from build123d import *

# Parameters (mm, degrees)
F0_W     = 945
F0_H     = 1805
F0_W_2   = 845
F0_H_2   = 1705
F1_DEPTH = 450
F2_W     = 945
F2_H     = 1805
F3_DEPTH = 1
F4_W     = 422.5
F4_H     = 50
F5_DEPTH = 350


with BuildPart() as f1:
    # F0 (on Front) → F1 (new body)
    with BuildSketch(Plane.XZ):
        Rectangle(F0_W, F0_H)
        Rectangle(F0_W_2, F0_H_2, mode=Mode.SUBTRACT)
    extrude(amount=F1_DEPTH)

    # F2 (on face) → F3 (join)
    with BuildSketch(Plane(origin=(0, 0, 0), x_dir=(-1, 0, 0), z_dir=(0, 1, 0))):
        Rectangle(F2_W, F2_H)
    extrude(amount=F3_DEPTH)

    # F4 (on face) → F5 (join)
    with BuildSketch(Plane.XZ):
        Polygon((422.5, 672.5), (-422.5, 672.5), (-422.5, 622.5), (0, 622.5), (50, 622.5), (422.5, 622.5), align=None)
        Polygon((50, 622.5), (0, 622.5), (0, 322.5), (0, 272.5), (0, -27.5), (0, -77.5), (0, -377.5), (0, -427.5), (0, -852.5), (50, -852.5), align=None)
        with Locations((-211.25, 297.5)):
            Rectangle(F4_W, F4_H)
        with Locations((-211.25, -52.5)):
            Rectangle(F4_W, F4_H)
        with Locations((-211.25, -402.5)):
            Rectangle(F4_W, F4_H)
    extrude(amount=F5_DEPTH)


solid = f1.part
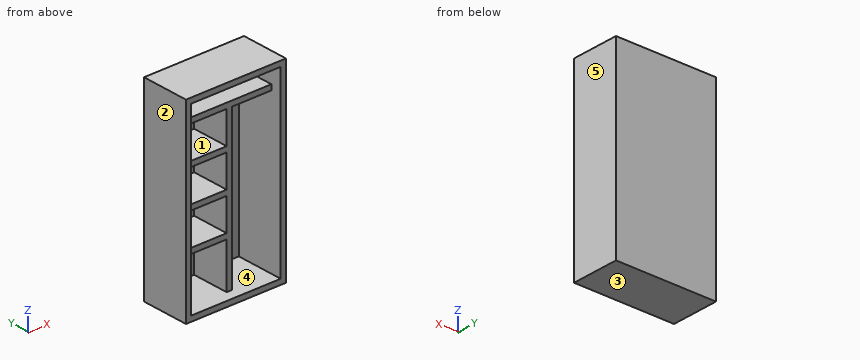
Check sheet for the modelled part. Datum: model origin and axes. Units: mm. Face numbers are marked on the shaded views. A direction names the side the tool comes from. Round coordinates to 2 decimals unless told otherwise and drop trailing zeros. Order: outer loops, then holes, each group sorted by start corner. A loop starts at its lowest first (then second) coordinate and runs counter-clockwise, first axis right, second up.
(1) Scan lines: probe 1 along X at (y, z) = (-209, 271); probe 2 along Z at (x, y) = (-131.5, -191); probe 3 along Z at (x, y) = (271.5, -257). Record each from-to range of solid material in increasing order.
(2) Cross-section at A-A, the plane y = -385. Enter the section's corners in (x, z).
(3) Go/stop test with a flat-tipped pin: P1, Ø8, axis at x = 71.5, z = 712, coming from the -Y side. Record where the tip stops, or that it passes through.
(4) Cross-section at C-C, the plane z = 693. Enter the section's corners in (x, y).
(5) Cross-section at D-D, the plane y = -95.5. Enter the section's corners in (x, z), and give its area (3 significant figures).
(6) Draft check along X on the marked faces 3, 4 and 5. Enter one of: pulls with the +X half, pulls with the -X half, needs draft (parallel to the pull), parting line crosses it, or undercut.
(7) Access from +Z, -Z, +X, -X, +Y, -Y to the whole of each face (thin tool, end or side, straight path). Record for the marked faces 1 and 2.
(8) Cross-section at B-B, the plane x = 392. Enter the section's corners in (y, z).
Check sheet entries:
1. probe 1: x = -472.5 to -422.5, 0 to 50, 422.5 to 472.5
1. probe 2: z = -902.5 to -852.5, -427.5 to -377.5, -77.5 to -27.5, 272.5 to 322.5, 622.5 to 672.5, 852.5 to 902.5
1. probe 3: z = -902.5 to -852.5, 622.5 to 672.5, 852.5 to 902.5
2. outline: (-472.5, -902.5) - (472.5, -902.5) - (472.5, 902.5) - (-472.5, 902.5) - close; hole (-422.5, -852.5) - (422.5, -852.5) - (422.5, 852.5) - (-422.5, 852.5) - close
3. P1: stops at y = 0
4. outline: (-472.5, -450) - (-422.5, -450) - (-422.5, 0) - (422.5, 0) - (422.5, -450) - (472.5, -450) - (472.5, 1) - (-472.5, 1) - close
5. outline: (-472.5, -902.5) - (472.5, -902.5) - (472.5, 902.5) - (-472.5, 902.5) - close; hole (-422.5, -852.5) - (0, -852.5) - (0, -427.5) - (-422.5, -427.5) - close; hole (-422.5, -377.5) - (0, -377.5) - (0, -77.5) - (-422.5, -77.5) - close; hole (-422.5, -27.5) - (0, -27.5) - (0, 272.5) - (-422.5, 272.5) - close; hole (-422.5, 322.5) - (0, 322.5) - (0, 622.5) - (-422.5, 622.5) - close; hole (-422.5, 672.5) - (422.5, 672.5) - (422.5, 852.5) - (-422.5, 852.5) - close; hole (50, -852.5) - (422.5, -852.5) - (422.5, 622.5) - (50, 622.5) - close
5. area: 444,000 mm2
6. face 3: needs draft
6. face 4: undercut
6. face 5: pulls with the +X half
7. face 1: -Y
7. face 2: +Z, -Z, -X, +Y, -Y
8. outline: (-450, -902.5) - (1, -902.5) - (1, 902.5) - (-450, 902.5) - (-450, 852.5) - (0, 852.5) - (0, 672.5) - (-350, 672.5) - (-350, 622.5) - (0, 622.5) - (0, -852.5) - (-450, -852.5) - close
